```python
from build123d import *

# Parameters (mm, degrees)
SKETCH1_W           = 95
SKETCH1_H           = 135
BOSS_EXTRUDE1_DEPTH = 65
CUT_EXTRUDE1_DEPTH  = 127
FILLET1_R           = 1


with BuildPart() as part:
    # Sketch1 → Boss-Extrude1 (new body)
    with BuildSketch(Plane(origin=(0, 0, 0), x_dir=(1, 0, 0), z_dir=(0, 1, 0))):
        Rectangle(SKETCH1_W, SKETCH1_H)
    extrude(amount=BOSS_EXTRUDE1_DEPTH)

    # Sketch2 → Cut-Extrude1 (cut)
    with BuildSketch(Plane.XY.offset(63.5)):
        with BuildLine():
            Line((-44.5, 25), (-44.5, 70))
            Line((-44.5, 70), (44.5, 70))
            Line((44.5, 70), (44.5, 25))
            ThreePointArc((44.5, 25), (22.5, 3), (0.5, 25))
            Line((0.5, 25), (-0.5, 25))
            ThreePointArc((-0.5, 25), (-22.5, 3), (-44.5, 25))
        make_face()
    extrude(amount=-CUT_EXTRUDE1_DEPTH, mode=Mode.SUBTRACT)

    # Fillet1
    # the kernel refuses this fillet: 1 mm, written as the material it takes off along each edge
    with BuildSketch(Plane(origin=(0.5, 25, 63.5), x_dir=(-1, 0, 0), z_dir=(0, 0, -1))) as fillet1_piece_1:
        with BuildLine():
            CenterArc((0.978250586, -1), FILLET1_R, 90, 87.508093631)
            ThreePointArc((-0.020803787, -0.956521739), (-0.005201562, -0.478373974), (0, 0))
            Line((0, 0), (0.978250586, 0))
        make_face()
    extrude(amount=127, mode=Mode.SUBTRACT)
    with BuildSketch(Plane(origin=(-0.5, 25, 63.5), x_dir=(-0.02174427153342351, -0.9997635653770749, 0), z_dir=(0, 0, -1))) as fillet1_piece_2:
        with BuildLine():
            CenterArc((0.978492219, -0.999763565), FILLET1_R, 91.245953184, 87.508093631)
            Line((-0.021271346, -0.978019294), (0, 0))
            ThreePointArc((0, 0), (0.478373974, -0.005201562), (0.956747947, 0))
        make_face()
    extrude(amount=127, mode=Mode.SUBTRACT)

    # Chamfer1
    # the kernel refuses this chamfer: 10 mm, written as the material it takes off along each edge
    with BuildSketch(Plane(origin=(-44.5, 65, 63.5), x_dir=(0, 0.027495876610586317, 0.9996219169112968), z_dir=(1, 0, 0))) as chamfer1_piece_1:
        with BuildLine():
            Line((10.286731952, 0), (-0.565471549, 10.271177935))
            Line((-0.565471549, 10.271177935), (-0.765395932, 10.26567876))
            ThreePointArc((-0.765395932, 10.26567876), (-0.341292271, 5.133978296), (-0.199924383, -0.005499175))
            Line((-0.199924383, -0.005499175), (0.005499175, -0.199924383))
            ThreePointArc((0.005499175, -0.199924383), (5.144976647, -0.058556496), (10.292231127, -0.199924383))
            Line((10.292231127, -0.199924383), (10.286731952, 0))
        make_face()
    extrude(amount=89, mode=Mode.SUBTRACT)
    with BuildSketch(Plane(origin=(44.5, 65, 63.5), x_dir=(0.9996219169112968, 0.027495876610586317, 0), z_dir=(0, 0, -1)), Plane(origin=(-44.5, 65, -63.5), x_dir=(-0.9996219169112968, 0.027495876610586317, 0), z_dir=(0, 0, 1))) as chamfer1_piece_2:
        with BuildLine():
            Line((10.286731952, 0), (-0.565471549, 10.271177935))
            Line((-0.565471549, 10.271177935), (-0.765395932, 10.26567876))
            ThreePointArc((-0.765395932, 10.26567876), (-0.341292271, 5.133978296), (-0.199924383, -0.005499175))
            Line((-0.199924383, -0.005499175), (0.005499175, -0.199924383))
            ThreePointArc((0.005499175, -0.199924383), (5.144976647, -0.058556496), (10.292231127, -0.199924383))
            Line((10.292231127, -0.199924383), (10.286731952, 0))
        make_face()
    extrude(amount=127, mode=Mode.SUBTRACT)
    with BuildSketch(Plane(origin=(-44.5, 65, -63.5), x_dir=(0, 0.027495876610586317, -0.9996219169112968), z_dir=(1, 0, 0))) as chamfer1_piece_3:
        with BuildLine():
            Line((10.286731952, 0), (-0.565471549, -10.271177935))
            Line((-0.565471549, -10.271177935), (-0.765395932, -10.26567876))
            ThreePointArc((-0.765395932, -10.26567876), (-0.341292271, -5.133978296), (-0.199924383, 0.005499175))
            Line((-0.199924383, 0.005499175), (0.005499175, 0.199924383))
            ThreePointArc((0.005499175, 0.199924383), (5.144976647, 0.058556496), (10.292231127, 0.199924383))
            Line((10.292231127, 0.199924383), (10.286731952, 0))
        make_face()
    extrude(amount=89, mode=Mode.SUBTRACT)
    with BuildSketch(Plane(origin=(-70.21682988, 65, 63.5), x_dir=(0, 0.027495876610586317, 0.9996219169112968), z_dir=(1, 0, 0))) as chamfer1_piece_4a_section:
        with BuildLine():
            Line((10.286731952, 0), (-0.565471549, 10.271177935))
            Line((-0.565471549, 10.271177935), (-0.765395932, 10.26567876))
            ThreePointArc((-0.765395932, 10.26567876), (-0.341292271, 5.133978296), (-0.199924383, -0.005499175))
            Line((-0.199924383, -0.005499175), (0.005499175, -0.199924383))
            ThreePointArc((0.005499175, -0.199924383), (5.144976647, -0.058556496), (10.292231127, -0.199924383))
            Line((10.292231127, -0.199924383), (10.286731952, 0))
        make_face()
    chamfer1_piece_4a = extrude(amount=114.71682988, mode=Mode.PRIVATE)
    chamfer1_piece_4a = split(chamfer1_piece_4a, bisect_by=Plane(origin=(-44.5, 61.702063732, 66.797936268), z_dir=(-1, 0, 0)), keep=Keep.TOP, mode=Mode.PRIVATE)
    with BuildSketch(Plane(origin=(-44.5, 65, -63.5), x_dir=(-0.9996219169112968, 0.027495876610586317, 0), z_dir=(0, 0, 1))) as chamfer1_piece_4b_section:
        with BuildLine():
            Line((10.286731952, 0), (-0.565471549, 10.271177935))
            Line((-0.565471549, 10.271177935), (-0.765395932, 10.26567876))
            ThreePointArc((-0.765395932, 10.26567876), (-0.341292271, 5.133978296), (-0.199924383, -0.005499175))
            Line((-0.199924383, -0.005499175), (0.005499175, -0.199924383))
            ThreePointArc((0.005499175, -0.199924383), (5.144976647, -0.058556496), (10.292231127, -0.199924383))
            Line((10.292231127, -0.199924383), (10.286731952, 0))
        make_face()
    chamfer1_piece_4b = extrude(amount=152.71682988, mode=Mode.PRIVATE)
    chamfer1_piece_4b = split(chamfer1_piece_4b, bisect_by=Plane(origin=(-47.797936268, 61.702063732, 63.5), z_dir=(0, 0, 1)), keep=Keep.TOP, mode=Mode.PRIVATE)
    chamfer1_piece_4 = chamfer1_piece_4a & chamfer1_piece_4b
    add(chamfer1_piece_4, mode=Mode.SUBTRACT)
    with BuildSketch(Plane(origin=(44.5, 65, 89.21682988), x_dir=(0.9996219169112968, 0.027495876610586317, 0), z_dir=(0, 0, -1))) as chamfer1_piece_5a_section:
        with BuildLine():
            Line((10.286731952, 0), (-0.565471549, 10.271177935))
            Line((-0.565471549, 10.271177935), (-0.765395932, 10.26567876))
            ThreePointArc((-0.765395932, 10.26567876), (-0.341292271, 5.133978296), (-0.199924383, -0.005499175))
            Line((-0.199924383, -0.005499175), (0.005499175, -0.199924383))
            ThreePointArc((0.005499175, -0.199924383), (5.144976647, -0.058556496), (10.292231127, -0.199924383))
            Line((10.292231127, -0.199924383), (10.286731952, 0))
        make_face()
    chamfer1_piece_5a = extrude(amount=152.71682988, mode=Mode.PRIVATE)
    chamfer1_piece_5a = split(chamfer1_piece_5a, bisect_by=Plane(origin=(47.797936268, 61.702063732, 63.5), z_dir=(0, 0, 1)), keep=Keep.TOP, mode=Mode.PRIVATE)
    with BuildSketch(Plane(origin=(-44.5, 65, 63.5), x_dir=(0, 0.027495876610586317, 0.9996219169112968), z_dir=(1, 0, 0))) as chamfer1_piece_5b_section:
        with BuildLine():
            Line((10.286731952, 0), (-0.565471549, 10.271177935))
            Line((-0.565471549, 10.271177935), (-0.765395932, 10.26567876))
            ThreePointArc((-0.765395932, 10.26567876), (-0.341292271, 5.133978296), (-0.199924383, -0.005499175))
            Line((-0.199924383, -0.005499175), (0.005499175, -0.199924383))
            ThreePointArc((0.005499175, -0.199924383), (5.144976647, -0.058556496), (10.292231127, -0.199924383))
            Line((10.292231127, -0.199924383), (10.286731952, 0))
        make_face()
    chamfer1_piece_5b = extrude(amount=114.71682988, mode=Mode.PRIVATE)
    chamfer1_piece_5b = split(chamfer1_piece_5b, bisect_by=Plane(origin=(44.5, 61.702063732, 66.797936268), z_dir=(1, 0, 0)), keep=Keep.TOP, mode=Mode.PRIVATE)
    chamfer1_piece_5 = chamfer1_piece_5a & chamfer1_piece_5b
    add(chamfer1_piece_5, mode=Mode.SUBTRACT)
    with BuildSketch(Plane(origin=(-44.5, 65, -63.5), x_dir=(0, 0.027495876610586317, -0.9996219169112968), z_dir=(1, 0, 0))) as chamfer1_piece_6a_section:
        with BuildLine():
            Line((10.286731952, 0), (-0.565471549, -10.271177935))
            Line((-0.565471549, -10.271177935), (-0.765395932, -10.26567876))
            ThreePointArc((-0.765395932, -10.26567876), (-0.341292271, -5.133978296), (-0.199924383, 0.005499175))
            Line((-0.199924383, 0.005499175), (0.005499175, 0.199924383))
            ThreePointArc((0.005499175, 0.199924383), (5.144976647, 0.058556496), (10.292231127, 0.199924383))
            Line((10.292231127, 0.199924383), (10.286731952, 0))
        make_face()
    chamfer1_piece_6a = extrude(amount=114.71682988, mode=Mode.PRIVATE)
    chamfer1_piece_6a = split(chamfer1_piece_6a, bisect_by=Plane(origin=(44.5, 61.702063732, -66.797936268), z_dir=(1, 0, 0)), keep=Keep.TOP, mode=Mode.PRIVATE)
    with BuildSketch(Plane(origin=(44.5, 65, 63.5), x_dir=(0.9996219169112968, 0.027495876610586317, 0), z_dir=(0, 0, -1))) as chamfer1_piece_6b_section:
        with BuildLine():
            Line((10.286731952, 0), (-0.565471549, 10.271177935))
            Line((-0.565471549, 10.271177935), (-0.765395932, 10.26567876))
            ThreePointArc((-0.765395932, 10.26567876), (-0.341292271, 5.133978296), (-0.199924383, -0.005499175))
            Line((-0.199924383, -0.005499175), (0.005499175, -0.199924383))
            ThreePointArc((0.005499175, -0.199924383), (5.144976647, -0.058556496), (10.292231127, -0.199924383))
            Line((10.292231127, -0.199924383), (10.286731952, 0))
        make_face()
    chamfer1_piece_6b = extrude(amount=152.71682988, mode=Mode.PRIVATE)
    chamfer1_piece_6b = split(chamfer1_piece_6b, bisect_by=Plane(origin=(47.797936268, 61.702063732, -63.5), z_dir=(0, 0, -1)), keep=Keep.TOP, mode=Mode.PRIVATE)
    chamfer1_piece_6 = chamfer1_piece_6a & chamfer1_piece_6b
    add(chamfer1_piece_6, mode=Mode.SUBTRACT)
    with BuildSketch(Plane(origin=(-70.21682988, 65, -63.5), x_dir=(0, 0.027495876610586317, -0.9996219169112968), z_dir=(1, 0, 0))) as chamfer1_piece_7a_section:
        with BuildLine():
            Line((10.286731952, 0), (-0.565471549, -10.271177935))
            Line((-0.565471549, -10.271177935), (-0.765395932, -10.26567876))
            ThreePointArc((-0.765395932, -10.26567876), (-0.341292271, -5.133978296), (-0.199924383, 0.005499175))
            Line((-0.199924383, 0.005499175), (0.005499175, 0.199924383))
            ThreePointArc((0.005499175, 0.199924383), (5.144976647, 0.058556496), (10.292231127, 0.199924383))
            Line((10.292231127, 0.199924383), (10.286731952, 0))
        make_face()
    chamfer1_piece_7a = extrude(amount=114.71682988, mode=Mode.PRIVATE)
    chamfer1_piece_7a = split(chamfer1_piece_7a, bisect_by=Plane(origin=(-44.5, 61.702063732, -66.797936268), z_dir=(-1, 0, 0)), keep=Keep.TOP, mode=Mode.PRIVATE)
    with BuildSketch(Plane(origin=(-44.5, 65, -89.21682988), x_dir=(-0.9996219169112968, 0.027495876610586317, 0), z_dir=(0, 0, 1))) as chamfer1_piece_7b_section:
        with BuildLine():
            Line((10.286731952, 0), (-0.565471549, 10.271177935))
            Line((-0.565471549, 10.271177935), (-0.765395932, 10.26567876))
            ThreePointArc((-0.765395932, 10.26567876), (-0.341292271, 5.133978296), (-0.199924383, -0.005499175))
            Line((-0.199924383, -0.005499175), (0.005499175, -0.199924383))
            ThreePointArc((0.005499175, -0.199924383), (5.144976647, -0.058556496), (10.292231127, -0.199924383))
            Line((10.292231127, -0.199924383), (10.286731952, 0))
        make_face()
    chamfer1_piece_7b = extrude(amount=152.71682988, mode=Mode.PRIVATE)
    chamfer1_piece_7b = split(chamfer1_piece_7b, bisect_by=Plane(origin=(-47.797936268, 61.702063732, -63.5), z_dir=(0, 0, -1)), keep=Keep.TOP, mode=Mode.PRIVATE)
    chamfer1_piece_7 = chamfer1_piece_7a & chamfer1_piece_7b
    add(chamfer1_piece_7, mode=Mode.SUBTRACT)


solid = part.part
```
Input: part model. Units: mm. Frame: model coordinates. A direction names the side the tool comes from. Round coordinates to 2 decimals unless told otherwise and drop trailing zeros. Loops run counter-clockwise (first coordinate to the right, second up) from the corner with the lowest first, then second, coordinate; pieces in that order, holes last. Notation, with made-up numbers: M -7,37 L 8,37 A16 cw 8,52 Z; hole C 40,-28 d3. An arc over 180 degrees is marked long. Answer in a Markdown table with one row per item. Add a question column.
1. Set-up query: faces 1 (the face through (-1, 29, 67.5)), 2 (the face through (-46, 56.5, -0.9)). Return all of +Z, -Z, +X, -X, +Y, -Y with unobstructed straight access to the full face (end or side cutting, diameter ignored); none if empty.
2. Section C-C (y = 32). Output: boundary loops of the cut face in (x, z), and give its area (3 significant figures).
3. Section D-D (x = 10). Output: boundary loops of the cut face in (y, z).
4. Mould query, pull axis Z, two halves, no side actions, for faces 3 (the face through (-1, 0, -1)), 4 (the face through (-1, 29, -67.5)), 5 (the face through (46, 56.5, 0.9)). Classes: released by +Z, released by -Z, zero draft, split by the parting line, or undercut.
5. Ray query, probe 1 along X at (y, z) = (25, -44); probe 2 along Z at (x, y) = (34, 54.5); probe 3 along X at (y, z) = (10.5, 56.5). Return the intervals inside material, ascending.
6. Contact query for a flat-ended pin moving along its axis: pin 1 (4 mm diameter, centred on x = 20, z = -5.5, fed in from +Y). Output: stop coordinate, or through.
7. Section B-B (z = 55). Output: boundary loops of the cut face in (x, y), and give its area (3 significant figures).
8. Section A-A (x = 22.5). Output: boundary loops of the cut face in (y, z), and give its area (3 significant figures).
Values follow:
| question | item | result |
|---|---|---|
| 1 | face 1 | +Z, +X, -X, +Y, -Y |
| 1 | face 2 | +Y |
| 2 | outline | M -47.5,-67.5 L 47.5,-67.5 L 47.5,67.5 L -47.5,67.5 Z; hole M -44.5,-63.5 L 44.5,-63.5 L 44.5,63.5 L -44.5,63.5 Z |
| 2 | area | 1,520 mm^2 |
| 3 | outline | M 0,-67.5 L 59,-67.5 L 55,-63.5 L 6.9,-63.5 L 6.9,63.5 L 55,63.5 L 59,67.5 L 0,67.5 Z |
| 4 | face 3 | zero draft |
| 4 | face 4 | released by -Z |
| 4 | face 5 | undercut |
| 5 | probe 1 | -47.5 to -44.5, 44.5 to 47.5 |
| 5 | probe 2 | -67.5 to -63.5, 63.5 to 67.5 |
| 5 | probe 3 | -47.5 to -39.05, -5.95 to 5.95, 39.05 to 47.5 |
| 6 | pin 1 | y = 3.47 |
| 7 | outline | M -47.5,0 L 47.5,0 L 47.5,58 L 44.5,55 L 44.5,25 A22 cw 0.52,24.04 A1 ccw 0,24.88 A1 ccw -0.52,24.04 A22 cw -44.5,25 L -44.5,55 L -47.5,58 Z |
| 7 | area | 1,040 mm^2 |
| 8 | outline | M 0,-67.5 L 59,-67.5 L 55,-63.5 L 3,-63.5 L 3,63.5 L 55,63.5 L 59,67.5 L 0,67.5 Z |
| 8 | area | 837 mm^2 |
